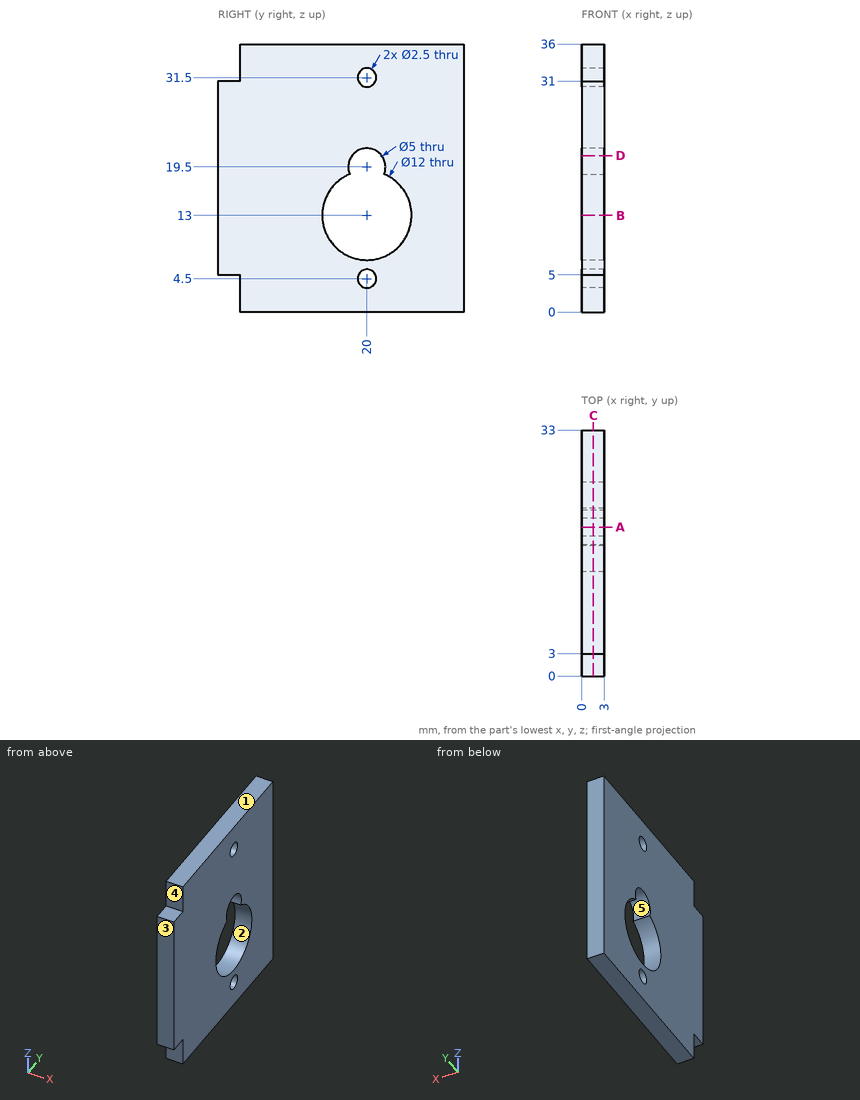
Design review of the part shown in the three views and the two pictorial views. Dimensions are in mm from the part's minimum x, y and z. A direction names the side the tool comes from. Round coordinates to 2 decimals unless told otherwise and drop trailing zeros. Write each loop counter-clockwise with the first axis right and the second up, starting at its lowest first coordinate (ties: lowest second). Pieces come first, ordered by that corner, then holes. Notation, with made-up numbers: M -14.5,12 L 40.5,12 A23 cw 40.5,23 Z; hole C 2.5,-37.5 d10. An arc over 180 degrees is marked long. One line per item, written item: value. Start each with the question number.
1. Take a section at B-B on z = 13. State the section outline as (x, y) points, then the cut area to 3 significant figures.
2. Take a section at A-A on y = 20. State the section outline as (x, z) points.
3. To check wall thickness, follow probe 1 along Z at (x, y) = (1.3, 20); probe 2 along Y at (x, z) = (1.65, 19.5); probe 3 along Y at (x, z) = (0.3, 13). State the ranges of each line that lie inside material, in increasing order. Write a range as from..to.
4. Take a section at C-C on x = 1.55. State the section outline as (y, z) points, then the cut area to 3 significant figures.
5. Clearance check with flat-ended pins moving along their axes: P1, Ø0.9, axis at x = 1.5, y = 1, coming from the -Z side; P2, Ø0.9, axis at x = 1.5, y = 1, coming from the +Z side. State where each tip first meets the part, or that it passes through.
6. For the marked faces 4 and 5, list the 3-axis set-ups (+Z, -Z, +X, -X, +Y, -Y) from which the entire face can be reached by the end or side of a thin tool; tool diameter is ignored.
7. Take a section at D-D on z = 21. State the section outline as (x, y) points.
8. Draft analysis for pull direction Z (two halves, no side actions). For the marked faces 1, 2 and 3, state which applies: pulls with the +Z half, pulls with the -Z half, needs draft (parallel to the pull), parting line crosses it, or undercut.
Computed:
1. outline: M 0,0 L 3,0 L 3,14 L 0,14 Z; M 0,26 L 3,26 L 3,33 L 0,33 Z
1. area: 63.0 mm²
2. outline: M 0,0 L 3,0 L 3,3.25 L 0,3.25 Z; M 0,5.75 L 3,5.75 L 3,7 L 0,7 Z; M 0,22 L 3,22 L 3,30.25 L 0,30.25 Z; M 0,32.75 L 3,32.75 L 3,36 L 0,36 Z
3. probe 1: z = 0..3.25, 5.75..7, 22..30.25, 32.75..36
3. probe 2: y = 0..17.5, 22.5..33
3. probe 3: y = 0..14, 26..33
4. outline: M 0,5 L 3,5 L 3,0 L 33,0 L 33,36 L 3,36 L 3,31 L 0,31 Z; hole M 17.69,18.54 A6 ccw long 22.31,18.54 A2.5 ccw long Z; hole C 20,4.5 d2.5; hole C 20,31.5 d2.5
4. area: 1,020 mm²
5. P1: stops at z = 5
5. P2: stops at z = 31
6. face 4: +Z, +X, -X, -Y
6. face 5: +X, -X
7. outline: M 0,0 L 3,0 L 3,18 L 0,18 Z; M 0,22 L 3,22 L 3,33 L 0,33 Z
8. face 1: pulls with the +Z half
8. face 2: undercut
8. face 3: needs draft
